Source: CAD feature listing. Evaluate the final solid. Frame: model axes, mm. A direction names the side the tool comes from. Coordinates: 2 decimals unless noted, no trailing zeros. Order: outer loops, then holes, each group sorted by start corner. A loop starts at its lowest first (then second) coordinate and runs counter-clockwise, first axis right, second up. Notation, with made-up numbers: (-34.75, -26) - (-18.75, -26) arc R4 ccw to (-18.75, -20) - close; hole circle Ø5 at (-13.5, -8). An arc over 180 degrees is marked (long way). One line per question, with ' | ' between items. Start each with the question number.
(1) Access query for faces 4 (the flat face through (-17, -6.525, 1)), 5 (the flat face through (12.75, -2, 1)), 6 (the flat face through (-14.75, 4, 2)). Directions: +Z, -Z, +X, -X, +Y, -Y. A direction counts if a zero-diameter tool reaches every point of the face in a straight line with its end or side. Return the directions, or none.
(2) Draft query along X for faces 1 (the flat face through (0, 3.675, 2)), 2 (the flat face through (-16, 1.175, 1)), 3 (the cylindrical face through (22.1, -2.76, 0.99)). Return one class per face: +X half, -X half, draft (parallel to the pull), parting line (faces both ways), or undercut.
(3) Section B-B (x = -4.7). Return the cut outline in (y, z) (3 decimals), then the cut area to 3 significant figures.
(4) Section A-A (y = 2.25). Return the cut outline in (x, z).
(5) Section D-D (y = -3.75). Return the cut outline in (x, z).
(6) Section C-C (z = 1.4). Return the cut outline in (x, y) (3 decimals), then the cut area to 3 significant figures.
(7) Contact query for flat-ended pins moving along their axis: P1, Ø0.6, axis at x = 16, z = 0.5, coming from the -Y side (3 decimals); P2, Ø2, axis at y = 3.5, z = 3, coming from the +X side; P3, Ø0.6, axis at y = 0.5, z = 1, coming from the +X side. Output: stop coordinate, or through.
(8) Line query: line 1 along Y through (x, z) = (18.25, 1.1) (3 decimals); line 2 along X through (y, z) = (3, 0.5); line 3 along X through (y, z) = (-1.5, 1.35). Output: solid intervals per line, ascending.
from build123d import *

# Parameters (mm, degrees)
SKETCH1_R           = 1.5
SKETCH1_W           = 25.5
SKETCH1_H           = 10.85
BOSS_EXTRUDE1_DEPTH = 2
SKETCH2_W           = 29.5
SKETCH2_H           = 2
BOSS_EXTRUDE2_DEPTH = 2.5
SKETCH3_R           = 1.7
BOSS_EXTRUDE3_DEPTH = 2.5


with BuildPart() as part:
    # Sketch1 → Boss-Extrude1 (new body)
    with BuildSketch(Plane.XY):
        with BuildLine():
            Line((-14.75, 5.675), (-14.75, 1.175))
            Line((-14.75, 1.175), (-18.25, 1.175))
            ThreePointArc((-18.25, 1.175), (-22.1, -2.675), (-18.25, -6.525))
            Line((-18.25, -6.525), (-14.75, -6.525))
            Line((-14.75, -6.525), (-14.75, -9.175))
            Line((-14.75, -9.175), (14.75, -9.175))
            Line((14.75, -9.175), (14.75, -6.525))
            Line((14.75, -6.525), (18.25, -6.525))
            ThreePointArc((18.25, -6.525), (22.1, -2.675), (18.25, 1.175))
            Line((18.25, 1.175), (14.75, 1.175))
            Line((14.75, 1.175), (14.75, 5.675))
            Line((14.75, 5.675), (-14.75, 5.675))
        make_face()
        with Locations((-18.25, -2.675)):
            Circle(SKETCH1_R, mode=Mode.SUBTRACT)
        with Locations(Location((18.25, -2.675, 0), (0, 0, 180))):
            Circle(SKETCH1_R, mode=Mode.SUBTRACT)
        with Locations((0, -1.75)):
            Rectangle(SKETCH1_W, SKETCH1_H, mode=Mode.SUBTRACT)
    extrude(amount=BOSS_EXTRUDE1_DEPTH)

    # Sketch2 → Boss-Extrude2 (add)
    with BuildSketch(Plane.XY.offset(2)):
        with Locations((0, 4.675)):
            Rectangle(SKETCH2_W, SKETCH2_H)
    extrude(amount=BOSS_EXTRUDE2_DEPTH)

    # Sketch3 → Boss-Extrude3 (add)
    with BuildSketch(Plane(origin=(0, 5.675, 0), x_dir=(1, 0, 0), z_dir=(0, 1, 0))):
        with Locations((-4.7, -2.25)):
            Circle(SKETCH3_R)
        with Locations((4.7, -2.25)):
            Circle(SKETCH3_R)
    extrude(amount=BOSS_EXTRUDE3_DEPTH)


solid = part.part
Response values:
1) face 4: +Z, -Z, -X, -Y | face 5: +Z, -Z | face 6: +Z, -Z, -X, +Y
2) face 1: undercut | face 2: draft | face 3: +X half
3) outline: (-9.175, 0) - (-7.175, 0) - (-7.175, 2) - (-9.175, 2) - close; (3.675, 0) - (5.675, 0) - (5.675, 0.55) - (8.175, 0.55) - (8.175, 3.95) - (5.675, 3.95) - (5.675, 4.5) - (3.675, 4.5) - close | area: 21.5 mm²
4) outline: (-14.75, 0) - (-12.75, 0) - (-12.75, 2) - (-14.75, 2) - close; (12.75, 0) - (14.75, 0) - (14.75, 2) - (12.75, 2) - close
5) outline: (-21.95, 0) - (-19.3, 0) - (-19.3, 2) - (-21.95, 2) - close; (-17.2, 0) - (-12.75, 0) - (-12.75, 2) - (-17.2, 2) - close; (12.75, 0) - (17.2, 0) - (17.2, 2) - (12.75, 2) - close; (19.3, 0) - (21.95, 0) - (21.95, 2) - (19.3, 2) - close
6) outline: (-18.25, -6.525) - (-14.75, -6.525) - (-14.75, -9.175) - (14.75, -9.175) - (14.75, -6.525) - (18.25, -6.525) arc R3.85 ccw to (18.25, 1.175) - (14.75, 1.175) - (14.75, 5.675) - (6.172, 5.675) - (6.172, 8.175) - (3.228, 8.175) - (3.228, 5.675) - (-3.228, 5.675) - (-3.228, 8.175) - (-6.172, 8.175) - (-6.172, 5.675) - (-14.75, 5.675) - (-14.75, 1.175) - (-18.25, 1.175) arc R3.85 ccw to start; hole circle Ø3 at (-18.25, -2.675); hole (-12.75, -7.175) - (12.75, -7.175) - (12.75, 3.675) - (-12.75, 3.675) - close; hole circle Ø3 at (18.25, -2.675) | area: 262 mm²
7) P1: stops at y = -6.525 | P2: stops at x = 14.75 | P3: stops at x = 20.81
8) line 1: y = -6.525 to -4.175, -1.175 to 1.175 | line 2: x = -14.75 to -12.75, 12.75 to 14.75 | line 3: x = -21.92 to -19.18, -17.32 to -12.75, 12.75 to 17.32, 19.18 to 21.92
